The drawing under review shows one solid part. Ordinate dimensions are in mm from its lowest x, y, z. Coordinates: 2 decimals unless noted, no trailing zeros. Loops run counter-clockwise (first coordinate to the right, second up) from the corner with the lowest first, then second, coordinate; pieces in that order, holes last. Notation, with made-up numbers: M -27.5,35 L -5.5,35 A30 ccw -5.5,63 Z; hole C -19,21.5 d1. An arc over 180 degrees is marked long. Use one line per item in the form item = value.
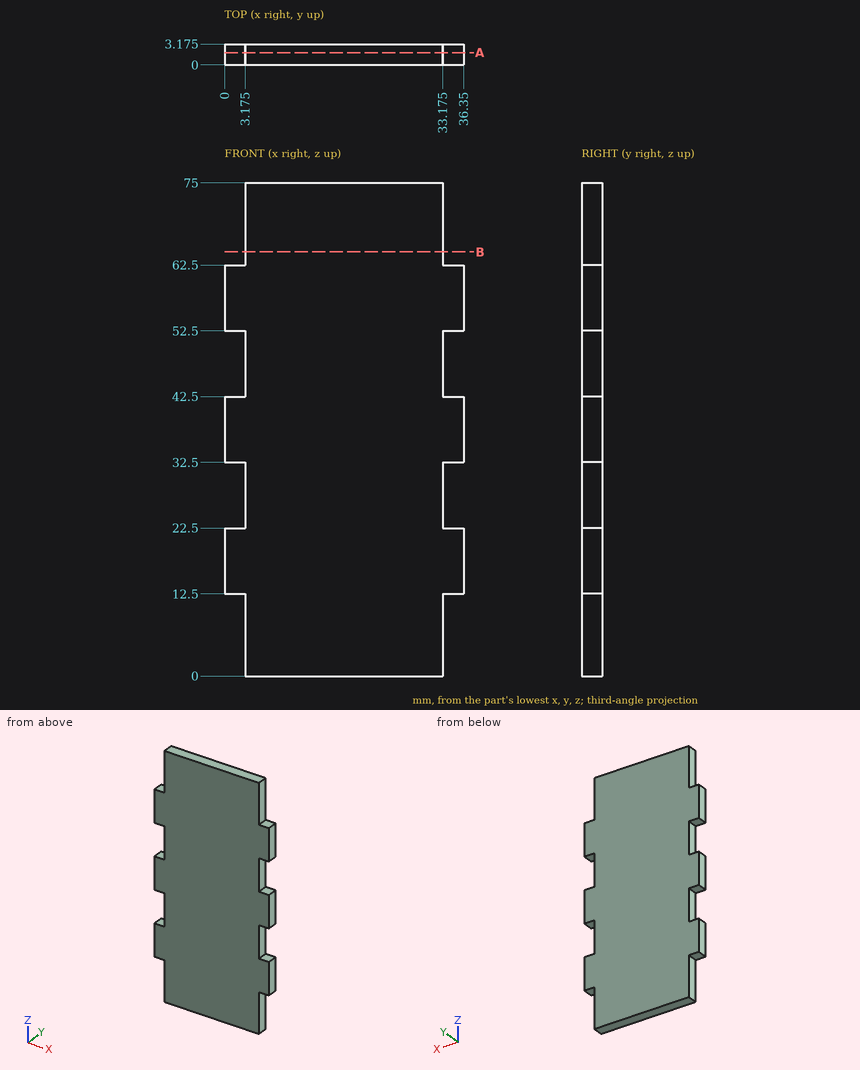
1. Consider section A-A on y = 1.85. Write out the cut boundary in (x, z) (3 decimals).
Computed values:
outline = M 0,12.5 L 3.175,12.5 L 3.175,0 L 33.175,0 L 33.175,12.5 L 36.35,12.5 L 36.35,22.5 L 33.175,22.5 L 33.175,32.5 L 36.35,32.5 L 36.35,42.5 L 33.175,42.5 L 33.175,52.5 L 36.35,52.5 L 36.35,62.5 L 33.175,62.5 L 33.175,75 L 3.175,75 L 3.175,62.5 L 0,62.5 L 0,52.5 L 3.175,52.5 L 3.175,42.5 L 0,42.5 L 0,32.5 L 3.175,32.5 L 3.175,22.5 L 0,22.5 Z
2. Consider section B-B on z = 64.5. Write out the cut boundary in (x, y) (3 decimals), plus the area to 4 significant figures.
Computed values:
outline = M 3.175,0 L 33.175,0 L 33.175,3.175 L 3.175,3.175 Z
area = 95.25 mm2
3. Wall thickness on line 1 along X through (y, z) = (2.5, 10.5) (3 decimals): over which ranges is the line inside the solid? List them lowest first. Write a range as from..to.
Computed values:
line_1 = 3.175..33.175
4. For pin 1 Ø1 at (x, y) = (1, 1.5) entering from -Z; pin 2 Ø1.5 at (y, z) = (1, 25) entering from +X (3 decimals); pin 3 Ø5 at (x, z) = (6, 23) entering from -Y; pin 4 Ø1.6 at (x, y) = (35.5, 1.5) entering from +Z, all flat-tipped, find the tip position at first contact; note any pin that passes through.
Computed values:
pin_1 = 12.5
pin_2 = 33.175
pin_3 = 0
pin_4 = 62.5
